from build123d import *

# Parameters (mm, degrees)
F1_DEPTH = 38
F3_DEPTH = 30.001
F4_R     = 2


with BuildPart() as f1:
    # F0 (on Front) → F1 (new body)
    with BuildSketch(Plane.XZ):
        Polygon((-2, 0), (0, 0), (0, 29.5), (26, 29.5), (26, 0), (28, 0), (28, 31.5), (-2, 31.5), align=None)
    extrude(amount=F1_DEPTH)

    # F2 (on face) → F3 (cut, through all)
    with BuildSketch(Plane(origin=(-2, 0, 0), x_dir=(0, -1, 0), z_dir=(-1, 0, 0))):
        with BuildLine():
            ThreePointArc((0, 0), (19, -19), (38, 0))
            Line((38, 0), (0, 0))
        make_face()
        with BuildLine():
            Line((0, 0), (38, 0))
            ThreePointArc((38, 0), (19, 19), (0, 0))
        make_face()
    extrude(amount=-F3_DEPTH, mode=Mode.SUBTRACT)

    # F4
    f4_edges = [f1.edges().sort_by_distance(p)[0] for p in [
        (26, -19, 29.5),
        (0, -19, 29.5),
        (28, -19, 31.5),
        (-2, -19, 31.5),
    ]]
    fillet(f4_edges, radius=F4_R)


solid = f1.part
Could you check a few things on this model? Use its own coordinates, in mm. A direction names the side the tool comes from. Round coordinates to 2 decimals unless told otherwise and drop trailing zeros. Write each loop counter-clockwise with the first axis right and the second up, starting at its lowest first coordinate (ties: lowest second). Pieces come first, ordered by that corner, then holes. Notation, with made-up numbers: (70, 52) - (102, 52) arc R29 ccw to (102, 74) - close; hole circle Ø8 at (24.5, 89). An arc over 180 degrees is marked (long way). Put each result on its own line as item: value. Start each with the question number.
(1) I want a section at B-B, the plane z = 28. Please give me the cut outline in (x, y), plus the area to 3 significant figures.
(2) Will this pin go through, and if not, where does the flat tip stop? pin 1 (1 mm diameter, centred on x = 14, y = -26, fed in from -Z).
(3) I need wall thicknesses on probe 1 along X at (y, z) = (-6, 21.5); probe 2 along Z at (x, y) = (22, -22.5); probe 3 along X at (y, z) = (-3, 28.5). Which ranges of each line are inside material? Lowest first, please.
(4) I want a section at D-D, the plane x = 3.25. Please give me the cut outline in (y, z).
(5) I want a section at A-A, the plane y = -19. Please give me the cut outline in (x, z), plus the area to 3 significant figures.
(6) For faces 5 (the cylindrical face through (25.4, -19.27, 28.93)), 6 (the cylindrical face through (27.43, -19.27, 30.9)), which set-ups out of +Z, -Z, +X, -X, +Y, -Y let a thin tool reach every point of the face, with its end or its side?
(7) Thinking about a two-plate mould opening in X: for faces 1 (the cylindrical face through (-1, -19, 19)), 2 (the flat face through (26, -19, 20)), 3 (the cylindrical face through (-1.4, -19.27, 30.93)), 4 (the flat face through (28, -19, 21)), which applies, released by +X, released by -X, zero draft, split by the parting line, or undercut?
(8) I want a section at C-C, the plane z = 8. Please give me the cut outline in (x, y).
Here are the results:
1. outline: (-2, -38) - (0.06, -38) - (0.06, 0) - (-2, 0) - close; (25.94, -38) - (28, -38) - (28, 0) - (25.94, 0) - close
1. area: 157 mm^2
2. pin 1: stops at z = 29.5
3. probe 1: x = -2 to 0, 26 to 28
3. probe 2: z = 29.5 to 31.5
3. probe 3: x = -2 to 0.27, 25.73 to 28
4. outline: (-38, 29.5) - (0, 29.5) - (0, 31.5) - (-38, 31.5) - close
5. outline: (-2, 19) - (0, 19) - (0, 27.5) arc R2 cw to (2, 29.5) - (24, 29.5) arc R2 cw to (26, 27.5) - (26, 19) - (28, 19) - (28, 29.5) arc R2 ccw to (26, 31.5) - (0, 31.5) arc R2 ccw to (-2, 29.5) - close
5. area: 102 mm^2
6. face 5: -Z, +Y, -Y
6. face 6: +Z, +X, +Y, -Y
7. face 1: zero draft
7. face 2: undercut
7. face 3: released by -X
7. face 4: released by +X
8. outline: (-2, -38) - (0, -38) - (0, -36.23) - (-2, -36.23) - close; (-2, -1.77) - (0, -1.77) - (0, 0) - (-2, 0) - close; (26, -38) - (28, -38) - (28, -36.23) - (26, -36.23) - close; (26, -1.77) - (28, -1.77) - (28, 0) - (26, 0) - close
